Verification items for the finished model (mm, model axes). Face numbers are marked on the shaded views. A direction names the side the tool comes from. Coordinates: 2 decimals unless noted, no trailing zeros. Write each loop counter-clockwise with the first axis right and the second up, starting at its lowest first coordinate (ties: lowest second). Pieces come first, ordered by that corner, then holes.
```python
from build123d import *


with BuildPart() as f1:
    # F0 (on Front) → F1 (revolve)
    with BuildSketch(Plane.XZ):
        Polygon((0, 8), (0, 0), (31.75, 0), (31.75, 8), (7.607925, 8), (4.185817, 8), align=None)
        Polygon((4.185817, 29.234255), (4.185817, 8), (7.607925, 8), (7.607925, 20.7), (33.007925, 20.7), (33.007925, 122.3), (28.189454, 122.3), (28.189454, 29.234255), align=None)
    revolve(axis=Axis((0, 0, 4), (0, 0, 1)))


solid = f1.part
```
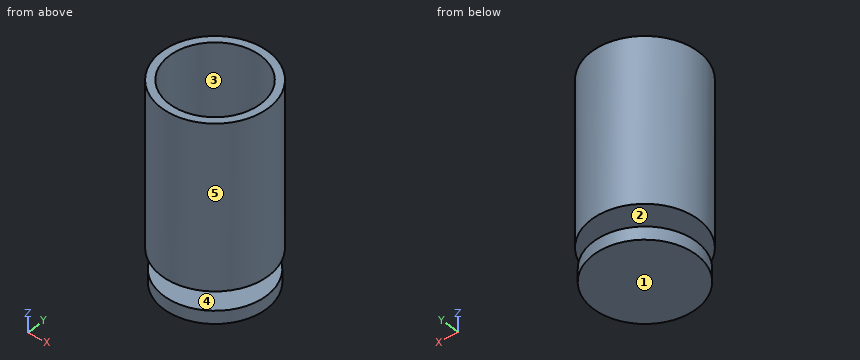
1. Sectioned sample at A-A, the plane y = 0. Record the boundary of the cut face in (x, z), and give its area (3 significant figures).
2. Gauge pin test, flat ends, axial feed: P1, Ø8, axis at x = 19.5, z = 78.5, coming from the -Y side; P2, Ø10, axis at y = 9, z = 106, coming from the +X side; P3, Ø1, axis at y = -13.5, z = 45.5, coming from the -X side. Record the tip position at first contact, or that the pin passes through.
3. Sectioned sample at B-B, the plane x = -11.5. Record the boundary of the cut face in (y, z).
4. Sectioned sample at C-C, the plane z = 59.5. Record the boundary of the cut face in (x, y).
5. Tool access check on the marked faces 4 and 5. Record the directions out of +Z, -Z, +X, -X, +Y, -Y that give a thin tool (end or side, any length) a straight path to the whole face; none if there is none.
6. Material ranges on L1, parallel to Z at x = 24, y = 0; L2, parallel to Y at x = 0, z = 71; L3, parallel to Z at x = 3.5, y = 30, recorded low to high.
7. Draft check along Z on the marked faces 1, 2 and 3. Enter one of: pulls with the +Z half, pulls with the -Z half, needs draft (parallel to the pull), parting line crosses it, or undercut.
Outcome:
1. outline: (-33.01, 20.7) - (-7.61, 20.7) - (-7.61, 8) - (-31.75, 8) - (-31.75, 0) - (31.75, 0) - (31.75, 8) - (7.61, 8) - (7.61, 20.7) - (33.01, 20.7) - (33.01, 122.3) - (28.19, 122.3) - (28.19, 29.23) - (4.19, 29.23) - (4.19, 8) - (-4.19, 8) - (-4.19, 29.23) - (-28.19, 29.23) - (-28.19, 122.3) - (-33.01, 122.3) - close
1. area: 1,980 mm2
2. P1: stops at y = -29.14
2. P2: stops at x = 32.76
2. P3: stops at x = -30.34
3. outline: (-30.94, 20.7) - (30.94, 20.7) - (30.94, 122.3) - (25.74, 122.3) - (25.74, 29.23) - (-25.74, 29.23) - (-25.74, 122.3) - (-30.94, 122.3) - close; (-29.59, 0) - (29.59, 0) - (29.59, 8) - (-29.59, 8) - close
4. outline: circle Ø66.02 at (0, 0); hole circle Ø56.38 at (0, 0)
5. face 4: none
5. face 5: +Z, -Z
6. L1: z = 0 to 8, 20.7 to 29.23
6. L2: y = -33.01 to -28.19, 28.19 to 33.01
6. L3: z = 0 to 8, 20.7 to 122.3
7. face 1: pulls with the -Z half
7. face 2: undercut
7. face 3: needs draft
